Autodesk Inventor part; units mm, degrees
ref_plane "YZ Plane" through (0, 0, 0) normal (1, 0, 0) x (0, 1, 0)
ref_plane "XZ Plane" through (0, 0, 0) normal (0, 1, 0) x (-1, 0, 0)
ref_plane "XY Plane" through (0, 0, 0) normal (0, 0, 1) x (1, 0, 0)
sketch "Sketch1" plane through (0, 0, 0) normal (0, 0, 1) x (1, 0, 0)
  line L0 (-6.35, -3.6662) -> (-6.35, 3.6662)
  line L1 (-6.35, 3.6662) -> (0, 7.3323)
  line L2 (0, 7.3323) -> (6.35, 3.6662)
  line L3 (6.35, 3.6662) -> (6.35, -3.6662)
  line L4 (6.35, -3.6662) -> (0, -7.3323)
  line L5 (0, -7.3323) -> (-6.35, -3.6662)
  point P0 (0, 0)
  point P1 (0, 0)
  dimension "Size" = 12.7
extrude "Extrusion1" add sketch "Sketch1" along normal mid plane 50.8
sketch "Sketch2" plane through (0, 0, 25.4) normal (0, 0, 1) x (1, 0, 0)
  line L0 (-6.35, 3.6662) -> (-6.35, -3.6662) construction
  line L1 (-6.35, -3.6662) -> (0, -7.3323) construction
  line L2 (0, -7.3323) -> (6.35, -3.6662) construction
  line L3 (6.35, -3.6662) -> (6.35, 3.6662) construction
  line L4 (6.35, 3.6662) -> (0, 7.3323) construction
  line L5 (0, 7.3323) -> (-6.35, 3.6662) construction
  circle A0 centre (0, 0) radius 6.35
extrude "Extrusion2" add sketch "Sketch2" along normal blind 7.9248
mirror "Mirror1" about plane through (0, 0, 0) normal (0, 0, 1) of "Extrusion2"
properties part number "SHAFT" material "Aluminum 6061"
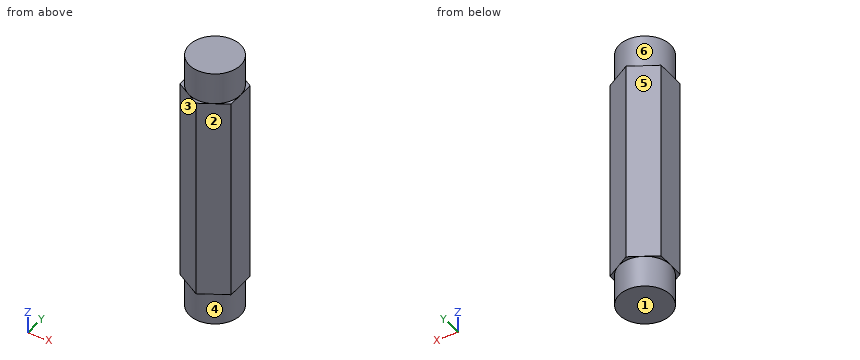
Read the model definition and answer for the solid it produces. Units are mm, in the model's axes. Face numbers are marked on the shaded views. A direction names the side the tool comes from. Coordinates: 2 decimals unless noted, no trailing zeros. Loops run counter-clockwise (first coordinate to the right, second up) from the corner with the lowest first, then second, coordinate; pieces in that order, holes last. Notation, with made-up numbers: (81.25, 58) -> (95.25, 58) arc R7 cw to (95.25, 62) -> close; hole circle Ø10 at (34, -20.5). An arc over 180 degrees is marked (long way). Answer in a Markdown table with one row per item.
Item 1: For a pull along X with two mould halves and no side action, classify the marked faces 1, 2 and 3 as released by +X, released by -X, zero draft, split by the parting line, or undercut.
Returned:
| item | result |
|---|---|
| face 1 | zero draft |
| face 2 | released by +X |
| face 3 | released by -X |
Item 2: A cutting plane is placed at A-A on x = 1.25. Determine the outline of the cut face in (y, z), plus the area to 3 significant figures.
Returned:
| item | result |
|---|---|
| outline | (-6.61, -25.4) -> (-6.23, -25.4) -> (-6.23, -33.32) -> (6.23, -33.32) -> (6.23, -25.4) -> (6.61, -25.4) -> (6.61, 25.4) -> (6.23, 25.4) -> (6.23, 33.32) -> (-6.23, 33.32) -> (-6.23, 25.4) -> (-6.61, 25.4) -> close |
| area | 869 mm^2 |
Item 3: A cutting plane is placed at D-D on z = 29.5. Determine the outline of the cut face in (x, y), plus the area to 3 significant figures.
Returned:
| item | result |
|---|---|
| outline | circle Ø12.7 at (0, 0) |
| area | 127 mm^2 |
Item 4: Each of these flat-tipped pins is pushed along its axis until it touches: P1, Ø4, axis at x = 1, z = 21.5, coming from the -Y side; P2, Ø2, axis at x = -3, z = -8.5, coming from the -Y side. Where does it stop, or does it pass through?
Returned:
| item | result |
|---|---|
| P1 | stops at y = -7.33 |
| P2 | stops at y = -6.18 |
Item 5: Straight lines are drawn through the part: line 1 along X through (y, z) = (4.25, 10.5); line 2 along Y through (x, z) = (2.75, -6.5); line 3 along X through (y, z) = (-2.75, 27). For each, find the intervals that lie inside material, in ascending order. Write a range as [from, to].
Returned:
| item | result |
|---|---|
| line 1 | x = [-5.34, 5.34] |
| line 2 | y = [-5.74, 5.74] |
| line 3 | x = [-5.72, 5.72] |
Item 6: A cutting plane is placed at B-B on z = -18. Determine the outline of the cut face in (x, y).
Returned:
| item | result |
|---|---|
| outline | (-6.35, -3.67) -> (0, -7.33) -> (6.35, -3.67) -> (6.35, 3.67) -> (0, 7.33) -> (-6.35, 3.67) -> close |
Item 7: For the marked faces 4, 5 and 6, determine the directions among +Z, -Z, +X, -X, +Y, -Y from which every point of the face is accessible in a straight line to the end or side of a thin tool.
Returned:
| item | result |
|---|---|
| face 4 | -Z |
| face 5 | +Z, -Z, -X, +Y |
| face 6 | +Z |
Item 8: A cutting plane is placed at C-C on x = -2.5. Determine the outline of the cut face in (y, z).
Returned:
| item | result |
|---|---|
| outline | (-5.89, -25.4) -> (-5.84, -25.4) -> (-5.84, -33.32) -> (5.84, -33.32) -> (5.84, -25.4) -> (5.89, -25.4) -> (5.89, 25.4) -> (5.84, 25.4) -> (5.84, 33.32) -> (-5.84, 33.32) -> (-5.84, 25.4) -> (-5.89, 25.4) -> close |
